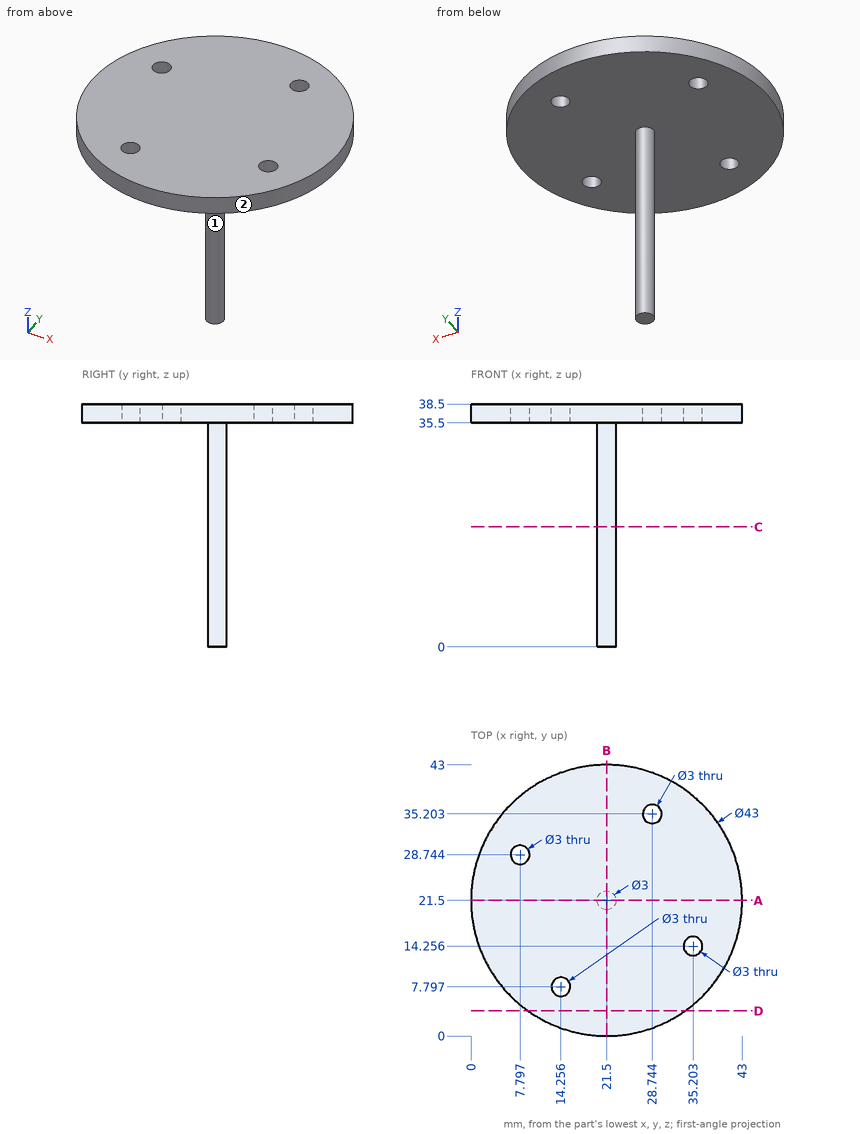
Job drawing, mm, ordinate dimensions from the low corner. One solid piece. A direction names the side the tool comes from. Coordinates: 2 decimals unless noted, no trailing zeros. Order: outer loops, then holes, each group sorted by start corner. A loop starts at its lowest first (then second) coordinate and runs counter-clockwise, first axis right, second up. Notation, with made-up numbers: M 30.25,-24 L 65.25,-24 A7 cw 65.25,-13 Z; hole C 88.5,64 d9. An arc over 180 degrees is marked long. Return JSON: item names as keys, results as strings.
1. Tool access for the marked faces 1 and 2: list every direction of +Z, -Z, +X, -X, +Y, -Y with a clear straight run to the whole face (end or side of a thin tool).
Ans:
{"face 1": "-Z", "face 2": "+Z, -Z"}
2. Saw through at C-C (z = 19). Give the cut face in (x, y), and give its area (3 significant figures).
Ans:
{"outline": "C 21.5,21.5 d3", "area": "7.07 mm^2"}
3. Saw through at A-A (y = 21.5). Give the cut face in (x, z).
Ans:
{"outline": "M 0,35.5 L 20,35.5 L 20,0 L 23,0 L 23,35.5 L 43,35.5 L 43,38.5 L 0,38.5 Z"}
4. Flat gauge pins, fed straight in: pin 1 (1.5 mm diameter, centred on x = 25, y = 8, fed in from -Z); pin 2 (4 mm diameter, centred on x = 20, z = 30, fed in from +Y). Where does each tip first touch, or does it go through?
Ans:
{"pin 1": "z = 35.5", "pin 2": "y = 23"}
5. Drill centre lines: probe 1 along Z at (x, y) = (22, 10.5); probe 2 along Y at (x, z) = (26, 37.5). Where is each one in solid material? Low to high.
Ans:
{"probe 1": "35.5 to 38.5", "probe 2": "0.48 to 42.52"}
6. Saw through at D-D (y = 4). Give the cut face in (x, z).
Ans:
{"outline": "M 9.01,35.5 L 33.99,35.5 L 33.99,38.5 L 9.01,38.5 Z"}
